Build history of the part. All positions in model axes, mm. A direction names the side the tool comes from. Round coordinates to 2 decimals unless told otherwise and drop trailing zeros. Write item = value, one per line.
from build123d import *
from build123d.topology import SkipClean

# Parameters (mm, degrees)
SKETCH_3_W          = 40
SKETCH_3_H          = 40
CUT_EXTRUDE_1_DEPTH = 70
CUT_REVOLVE_1_ANGLE = 90
CUT_EXTRUDE_2_DEPTH = 456.68629575
EXTRUDE_1_DEPTH     = 42
SKETCH_7_R          = 10
CUT_EXTRUDE_3_DEPTH = 440


with BuildPart() as part:
    # 草图1 → 旋转3 (revolve)
    with SkipClean():  # the faces are left unmerged after this step: merging them gives an invalid solid
        with BuildSketch(Plane(origin=(0, 0, 0), x_dir=(1, 0, 0), z_dir=(0, 1, 0))):
            with BuildLine():
                add(Edge.make_bspline(
                    [(200, 0), (200, 125), (0, 125), (-200, 125), (-200, 0)],
                    knots=[0, 0, 0, 1.570796327, 1.570796327, 3.141592654, 3.141592654, 3.141592654], degree=2, weights=[1, 0.707106781, 1, 0.707106781, 1]))
                Line((-200, 0), (200, 0))
            make_face()
            with BuildLine():
                Line((200, 0), (-200, 0))
                add(Edge.make_bspline(
                    [(-200, 0), (-200, -125), (0, -125), (200, -125), (200, 0)],
                    knots=[3.141592654, 3.141592654, 3.141592654, 4.71238898, 4.71238898, 6.283185307, 6.283185307, 6.283185307], degree=2, weights=[1, 0.707106781, 1, 0.707106781, 1]))
            make_face()
        revolve(axis=Axis((-376.776806715, 0, 0), (1, 0, 0)))
    add(part.part.scale(1), mode=Mode.REPLACE)  # the faces are merged on a copy

    # Surface Cut 1
    split(bisect_by=Plane.XY, keep=Keep.BOTTOM)

    # 草图3 → 切除-拉伸1 (cut)
    with BuildSketch(Plane(origin=(0, -125.246294878, -45.585923288), x_dir=(1, 0, 0), z_dir=(0, 0.9396926207859081, 0.34202014332566943))):
        with Locations((0, 43.622733675)):
            Rectangle(SKETCH_3_W, SKETCH_3_H)
    extrude(amount=CUT_EXTRUDE_1_DEPTH, mode=Mode.SUBTRACT)

    # 草图4 → 切除-旋转1 (revolve, cut)
    with BuildSketch(Plane.XY):
        with BuildLine():
            Line((-189.264857791, 10), (189.264857791, 10))
            add(Edge.make_bspline(
                [(189.264857791, 10), (189.01661408, 11.685645813), (188.399842232, 15.02459428), (186.660672029, 21.717695752), (183.544014825, 30.028723701), (178.280438028, 39.871100011), (169.238112825, 52.698753606), (154.190025082, 67.938441209), (130.617285564, 84.133702491), (102.331625356, 97.503941795), (70.346299789, 107.469826997), (35.819572857, 113.615740598), (0, 115.692129701), (-35.819572857, 113.615740598), (-70.346299789, 107.469826997), (-102.331625356, 97.503941795), (-130.617285564, 84.133702491), (-154.190025082, 67.938441209), (-169.238112825, 52.698753606), (-178.280438028, 39.871100011), (-183.544014825, 30.028723701), (-186.660672029, 21.717695752), (-188.399842232, 15.02459428), (-189.01661408, 11.685645813), (-189.264857791, 10)],
                knots=[0.091784635, 0.091784635, 0.091784635, 0.091784635, 0.13800375, 0.184222866, 0.276661096, 0.369099327, 0.461537558, 0.646414019, 0.831290481, 1.016166942, 1.201043404, 1.385919865, 1.570796327, 1.755672788, 1.94054925, 2.125425711, 2.310302173, 2.495178634, 2.680055096, 2.772493326, 2.864931557, 2.957369788, 3.003588903, 3.049808019, 3.049808019, 3.049808019, 3.049808019], degree=3))
        make_face()
    revolve(axis=Axis((-200, 0, 0), (-1, 0, 0)), revolution_arc=CUT_REVOLVE_1_ANGLE, mode=Mode.SUBTRACT)

    # 草图5 → 切除-拉伸2 (cut, through all)
    with BuildSketch(Plane(origin=(220, 0, 0), x_dir=(0, 0, -1), z_dir=(1, 0, 0))):
        with BuildLine():
            ThreePointArc((20, 20), (40, 0), (20, -20))
            Line((20, -20), (0, -20))
            Line((0, -20), (0, 20))
            Line((0, 20), (20, 20))
        make_face()
    extrude(amount=-CUT_EXTRUDE_2_DEPTH, mode=Mode.SUBTRACT)

    # 草图6 → 凸台-拉伸1 (add)
    with BuildSketch(Plane(origin=(220, 0, 0), x_dir=(0, 0, -1), z_dir=(1, 0, 0))):
        with BuildLine():
            Line((20, -20), (0, -20))
            Line((0, -20), (0, 20))
            Line((0, 20), (20, 20))
            ThreePointArc((20, 20), (40, 0), (20, -20))
        make_face()
    extrude_1 = extrude(amount=-EXTRUDE_1_DEPTH)

    # 镜向1: 凸台-拉伸1 across plane
    add(extrude_1.mirror(Plane(origin=(0, 0, 0), x_dir=(0, 0, 1), z_dir=(1, 0, 0))))

    # 草图7 → 切除-拉伸3 (cut)
    with BuildSketch(Plane(origin=(220, 0, 0), x_dir=(0, 0, -1), z_dir=(1, 0, 0))):
        with Locations((20, 0)):
            Circle(SKETCH_7_R)
    extrude(amount=-CUT_EXTRUDE_3_DEPTH, mode=Mode.SUBTRACT)


solid = part.part
1. Flat gauge pins, fed straight in: pin 1 (2 mm diameter, centred on x = 52.5, z = -62, fed in from -Y); pin 2 (4.5 mm diameter, centred on x = 183, z = -8.5, fed in from +Y); pin 3 (2.5 mm diameter, centred on x = -180.5, z = -6.5, fed in from +Y); pin 4 (8 mm diameter, centred on x = -67.5, y = -52.5, fed in from +Z). Where does each tip first touch, or does it go through?
Responses:
pin_1 = -104.09
pin_2 = 52.85
pin_3 = 55.07
pin_4 = 0
2. Probe probe 1 along Y at (x, z) = (-205, -20); probe 2 along Y at (x, z) = (23, -95.5); probe 3 along X at (y, z) = (-46.5, -81). List the from-to ranges inside material, lowest first.
Responses:
probe_1 = -20 to -10, 10 to 20
probe_2 = -79.36 to 0, 62.52 to 79.36
probe_3 = -132.92 to -20, 20 to 132.92
3. Mould opens along Z. For faces 4 (the face through (208, 20, -10)), 5 (the face through (-0.28, -44.45, -62.9)), 6 (the face through (-205, 0, -40)) say: pulls with the +Z half, pulls with the -Z half, needs draft (parallel to the pull), parting line crosses it, or undercut.
Responses:
face_4 = needs draft
face_5 = undercut
face_6 = pulls with the -Z half
4. Tool access for faces 1 (the face through (-0.28, -58.82, -89.114)), 2 (the face through (-179.72, 18.55, -27.48)), 3 (the face through (-178, 0, -7)): list every direction of +Z, -Z, +X, -X, +Y, -Y with a clear straight run to the whole face (end or side of a thin tool).
Responses:
face_1 = -Y
face_2 = none
face_3 = +Z
